Read the model definition and answer for the solid it produces. Units are mm, in the model's axes. Face numbers are marked on the shaded views. A direction names the side the tool comes from. Give positions to 0.01 mm unless a question says otherwise; leave off trailing zeros. Loops run counter-clockwise (first coordinate to the right, second up) from the corner with the lowest first, then second, coordinate; pieces in that order, holes last. Notation, with made-up numbers: (81, 64.25) -> (123, 64.25) arc R24 ccw to (123, 94.25) -> close; hole circle Ø8 at (84.5, 72.5). An arc over 180 degrees is marked (long way). Write each question's results on one line, items separated by ' | '. Start each with the question number.
Item 1: Find the intervals of material crossed by line 1 (Y direction, x = 4, z = -14); line 2 (Z direction, x = -8.5, y = -54.5); line 3 (Z direction, x = -33.5, y = -16), in increasing order.
Item 2: Section D-D on x = -57 is taken. Write down the section's boundary in (y, z).
Item 3: Section A-A on y = -18.75 is taken. Write down the section's boundary in (x, z).
Item 4: Section B-B on x = 7 is taken. Write down the section's boundary in (y, z), and give its area (3 significant figures).
Item 5: Which of the six approach directions +Z, -Z, +X, -X, +Y, -Y give full straight-line access (tool end or side, diameter ignored) to the marked faces 1, 2, 3 and 4?
Item 6: Each of these flat-tipped pins is pushed along its axis until it touches: P1, Ø4.5, axis at y = -65, z = 9, coming from the +X side; P2, Ø5, axis at x = -36, y = -103.5, coming from the -Z side; P3, Ø6, axis at y = -119.5, z = 14, coming from the +X side; P4, Ø4, axis at x = -43.56, y = -56.25, coming from the -Z side. Where does it stop, or does it pass through?
Item 7: Determine the mould class of the marked faces 5, 6 and 7 for opening direction X: +X half, -X half, draft (parallel to the pull), parting line (faces both ways), or undercut.
Item 8: Section C-C on z = 11 is taken. Write down the section's boundary in (x, y), and give its area (3 significant figures).
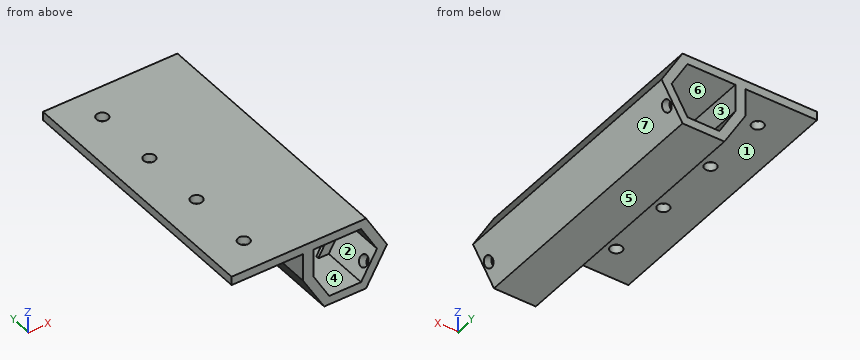
```python
from build123d import *

# Parameters (mm, degrees)
BOSS_EXTRUDE3_DEPTH = 150
SKETCH5_R           = 3.2639
CUT_EXTRUDE1_DEPTH  = 10
SKETCH6_R           = 3.15
CUT_EXTRUDE3_DEPTH  = 10
SKETCH7_W           = 23.443423468
SKETCH7_H           = 1.599424748
SKETCH7_H_2         = 1.6
BOSS_EXTRUDE4_DEPTH = 10


with BuildPart() as part:
    # Sketch4 → Boss-Extrude3 (new body)
    with BuildSketch(Plane(origin=(0, 0, 0), x_dir=(1, 0, 0), z_dir=(0, 1, 0))):
        Polygon((-23.557392252, 0.002600275), (-23.557392252, -15.452600275), (-63.557392252, -15.452600275), (-63.557392252, -20.302600275), (11.721711734, -20.302600275), (23.443423468, 0), (11.721711734, 20.302600275), (-11.721711734, 20.302600275), align=None)
        Polygon((-17.811255804, 0.05), (-17.811255804, -15.45), (8.920061659, -15.45), (17.840123318, 0), (8.920061659, 15.45), (-8.920061659, 15.45), align=None, mode=Mode.SUBTRACT)
    extrude(amount=-BOSS_EXTRUDE3_DEPTH)

    # Sketch5 → Cut-Extrude1 (cut)
    with BuildSketch(Plane(origin=(0, 0, 15.452600275), x_dir=(-1, 0, 0), z_dir=(0, 0, -1))):
        with Locations((43.557392252, -131.25)):
            Circle(SKETCH5_R)
        with Locations((43.557392252, -93.75)):
            Circle(SKETCH5_R)
        with Locations((43.557392252, -56.25)):
            Circle(SKETCH5_R)
        with Locations((43.557392252, -18.75)):
            Circle(SKETCH5_R)
    extrude(amount=-CUT_EXTRUDE1_DEPTH, mode=Mode.SUBTRACT)

    # Sketch6 → Cut-Extrude3 (cut)
    with BuildSketch(Plane(origin=(17.582567601, 0, -10.151300137), x_dir=(-0.4999999999999999, 0, -0.8660254037844387), z_dir=(0.8660254037844387, 0, -0.4999999999999999))):
        with Locations((0, -4.15)):
            Circle(SKETCH6_R)
        with Locations((0, -145.85)):
            Circle(SKETCH6_R)
    extrude(amount=-CUT_EXTRUDE3_DEPTH, mode=Mode.SUBTRACT)

    # Sketch7 → Boss-Extrude4 (add)
    with BuildSketch(Plane(origin=(17.582567601, 0, -10.151300137), x_dir=(-0.4999999999999999, 0, -0.8660254037844387), z_dir=(0.8660254037844387, 0, -0.4999999999999999))):
        with Locations((0, -26.499712374)):
            Rectangle(SKETCH7_W, SKETCH7_H)
        with Locations((0, -123.5)):
            Rectangle(SKETCH7_W, SKETCH7_H_2)
    extrude(amount=-BOSS_EXTRUDE4_DEPTH)


solid = part.part
```
Findings:
1) line 1: -124.3 to -122.7, -27.3 to -25.7 | line 2: -20.3 to -15.45, 15.45 to 20.3 | line 3: 15.45 to 20.3
2) outline: (-150, 15.45) -> (0, 15.45) -> (0, 20.3) -> (-150, 20.3) -> close
3) outline: (-63.56, 15.45) -> (-46.82, 15.45) -> (-46.82, 20.3) -> (-63.56, 20.3) -> close; (-40.29, 15.45) -> (-23.56, 15.45) -> (-23.56, 0) -> (-11.72, -20.3) -> (11.72, -20.3) -> (23.44, 0) -> (11.72, 20.3) -> (-40.29, 20.3) -> close; hole (-17.81, -0.05) -> (-8.92, -15.45) -> (8.92, -15.45) -> (17.84, 0) -> (8.92, 15.45) -> (-17.81, 15.45) -> close
4) outline: (-150, -20.3) -> (0, -20.3) -> (0, -15.45) -> (-25.7, -15.45) -> (-25.7, -8.48) -> (-27.3, -8.48) -> (-27.3, -15.45) -> (-122.7, -15.45) -> (-122.7, -8.48) -> (-124.3, -8.48) -> (-124.3, -15.45) -> (-150, -15.45) -> close; (-150, 15.45) -> (0, 15.45) -> (0, 20.3) -> (-150, 20.3) -> close | area: 1,480 mm2
5) face 1: -Z, -X, +Y, -Y | face 2: -Y | face 3: +Y, -Y | face 4: none
6) P1: x = 19.55 | P2: z = 15.45 | P3: x = 17.09 | P4: through
7) face 5: draft | face 6: undercut | face 7: +X half
8) outline: (-23.56, -150) -> (-17.81, -150) -> (-17.81, 0) -> (-23.56, 0) -> close; (11.49, -150) -> (17.09, -150) -> (17.09, 0) -> (11.49, 0) -> close | area: 1,700 mm2
